For this review, take the finished solid that the model builds, in its own axes (mm). Face numbers are marked on the shaded views. A direction names the side the tool comes from. Give positions to 0.01 mm unless a question says otherwise; leave off trailing zeros. Write each loop counter-clockwise with the first axis right and the second up, starting at its lowest first coordinate (ties: lowest second). Pieces come first, ordered by that corner, then holes.
1) We need section A-A on z = 0. Give the boundary of the cut face in (x, y).
2) We need section B-B on x = -132. Give the boundary of the cut face in (y, z).
3) Machinability: for the marked faces 1, 2, 3, 4 and 5, which of the approach directions +Z, -Z, +X, -X, +Y, -Y give a long, thin tool a straight path to every point of the face, cutting with its end or side? Answer none if there is none.
4) For P1, Ø4, axis at x = -94.5, y = 10.5, coming from the -Z side; P2, Ø1, axis at x = -133.5, y = 7, coming from the +Z side; P3, Ø3, axis at x = -118, y = -7, coming from the +Z side (3 decimals); P4, Ø20, axis at y = 2.5, z = 2, coming from the +X side, all flat-tipped, find the tip position at first contact; note any pin that passes through.
5) Wall thickness on line 1 along X through (y, z) = (11.5, 1); line 2 along Z through (x, y) = (-130, 0); line 3 along X through (y, z) = (-12.5, -5): over which ranges is each line inside the solid? List them lowest first.
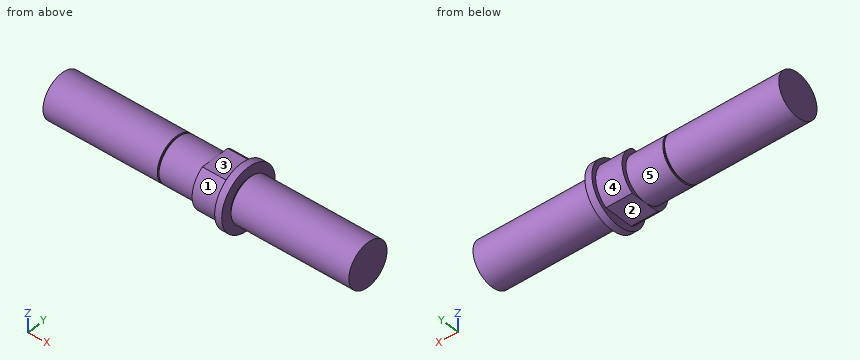
from build123d import *

# Parameters (mm, degrees)
SKETCH3_W          = 1
SKETCH3_H          = 1
SKETCH5_OUTSIDE_W  = 73.18
SKETCH5_OUTSIDE_H  = 73.18
CUT_EXTRUDE1_DEPTH = 15


with BuildPart() as part:
    # Sketch2 → Revolve1 (revolve)
    with BuildSketch(Plane.XY, mode=Mode.PRIVATE) as revolve1_sk:
        Polygon((0, 0), (0, 12.5), (-68, 12.5), (-68, 17.5), (-72, 17.5), (-72, 15), (-87, 15), (-87, 12.5), (-174, 12.5), (-174, 0), align=None)
    revolve(revolve1_sk.sketch.rotate(Axis((-174, 0, 0), (1, 0, 0)), 180), axis=Axis((-174, 0, 0), (1, 0, 0)))

    # Sketch3 → Cut-Revolve1 (revolve, cut)
    with BuildSketch(Plane.XY, mode=Mode.PRIVATE) as cut_revolve1_sk:
        with Locations((-67.5, 12)):
            Rectangle(SKETCH3_W, SKETCH3_H)
        with Locations((-108.5, 12)):
            Rectangle(SKETCH3_W, SKETCH3_H)
    revolve(cut_revolve1_sk.sketch.rotate(Axis((0, 0, 0), (-1, 0, 0)), 180), axis=Axis((0, 0, 0), (-1, 0, 0)), mode=Mode.SUBTRACT)

    # Sketch5 outside → Cut-Extrude1 (cut)
    with BuildSketch(Plane.ZY.offset(87)):
        Rectangle(SKETCH5_OUTSIDE_W, SKETCH5_OUTSIDE_H)
        with BuildLine():
            Line((-12.5, 8.291561976), (-12.5, -8.291561976))
            ThreePointArc((-12.5, -8.291561976), (0, -15), (12.5, -8.291561976))
            Line((12.5, -8.291561976), (12.5, 8.291561976))
            ThreePointArc((12.5, 8.291561976), (0, 15), (-12.5, 8.291561976))
        make_face(mode=Mode.SUBTRACT)
    extrude(amount=-CUT_EXTRUDE1_DEPTH, mode=Mode.SUBTRACT)


solid = part.part
Results list:
1. outline: (-174, -12.5) - (-109, -12.5) - (-109, -11.5) - (-108, -11.5) - (-108, -12.5) - (-87, -12.5) - (-87, -15) - (-72, -15) - (-72, -17.5) - (-68, -17.5) - (-68, -11.5) - (-67, -11.5) - (-67, -12.5) - (0, -12.5) - (0, 12.5) - (-67, 12.5) - (-67, 11.5) - (-68, 11.5) - (-68, 17.5) - (-72, 17.5) - (-72, 15) - (-87, 15) - (-87, 12.5) - (-108, 12.5) - (-108, 11.5) - (-109, 11.5) - (-109, 12.5) - (-174, 12.5) - close
2. outline: circle Ø25 at (0, 0)
3. face 1: -X, -Y
3. face 2: -Z, -X, +Y, -Y
3. face 3: +Z, -X, +Y, -Y
3. face 4: -X, +Y
3. face 5: -X
4. P1: stops at z = -9.17
4. P2: stops at z = 10.68
4. P3: stops at z = 11.225
4. P4: stops at x = 0
5. line 1: x = -174 to -109, -108 to -68, -67 to 0
5. line 2: z = -12.5 to 12.5
5. line 3: x = -87 to -68
